Check sheet for the drawn part. Datum: minimum x, y, z corner. Units: mm. A direction names the side the tool comes from. Coordinates: 2 decimals unless noted, no trailing zeros. Write each loop counter-clockwise with the first axis right and the second up, starting at its lowest first coordinate (ties: lowest second). Pieces come first, ordered by that corner, then holes. Notation, with made-up numbers: (1, 13) - (22, 13) arc R35 cw to (22, 45) - close; hole circle Ø10 at (-5, 11.5). An arc over 180 degrees is marked (long way). Write each question's results on one line, items separated by ' | '.
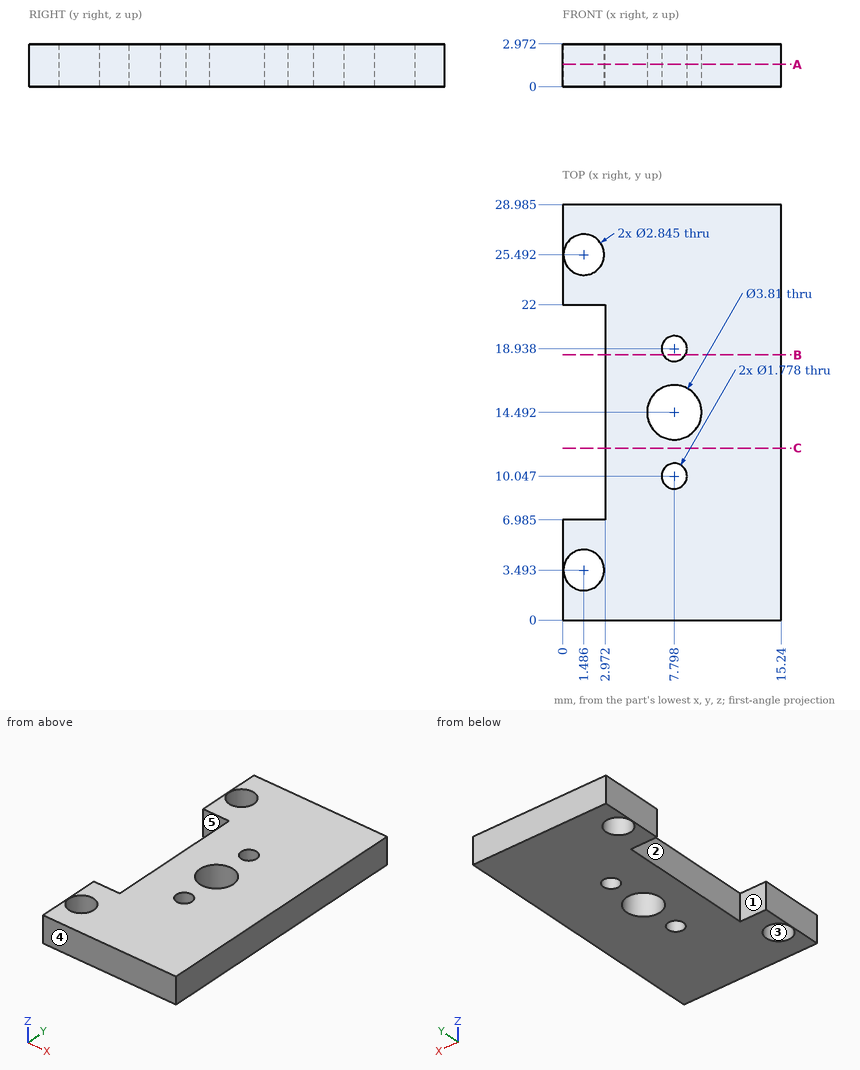
1. Access from +Z, -Z, +X, -X, +Y, -Y to the whole of each face (thin tool, end or side, straight path). Record for the marked faces 4 and 5.
Values follow:
face 4: +Z, -Z, +X, -X, -Y | face 5: +Z, -Z, -X
2. Sectioned sample at A-A (z = 1.55). Record the cut outline in (x, y) (1 decimal), then the cut area to 3 significant figures.
Values follow:
outline: (0, 0) - (15.2, 0) - (15.2, 29) - (0, 29) - (0, 22) - (3, 22) - (3, 7) - (0, 7) - close; hole circle Ø2.8 at (1.5, 3.5); hole circle Ø2.8 at (1.5, 25.5); hole circle Ø3.8 at (7.8, 14.5); hole circle Ø1.8 at (7.8, 10); hole circle Ø1.8 at (7.8, 18.9) | area: 368 mm^2
3. Draft check along X on the marked faces 1, 2 and 3. Enter one of: pulls with the +X half, pulls with the -X half, needs draft (parallel to the pull), parting line crosses it, or undercut.
Values follow:
face 1: needs draft | face 2: pulls with the -X half | face 3: undercut
4. Material ranges on L1, parallel to X at y = 21.5, z = 2.1; L2, parallel to Y at x = 1.25, z = 2.75 (1 decimal); L3, parallel to X at y = 19.25, z = 0.7 (1 decimal), recorded low to high. Write a range as [from, to].
Values follow:
L1: x = [2.97, 15.24] | L2: y = [0, 2.1], [4.9, 7], [22, 24.1], [26.9, 29] | L3: x = [3, 7], [8.6, 15.2]
5. Sectioned sample at B-B (y = 18.5). Record the cut outline in (x, z).
Values follow:
outline: (2.97, 0) - (7.02, 0) - (7.02, 2.97) - (2.97, 2.97) - close; (8.57, 0) - (15.24, 0) - (15.24, 2.97) - (8.57, 2.97) - close
6. Sectioned sample at C-C (y = 12). Record the cut outline in (x, z).
Values follow:
outline: (2.97, 0) - (15.24, 0) - (15.24, 2.97) - (2.97, 2.97) - close
